Model file for the job. Use its own axes, mm. A direction names the side the tool comes from. Coordinates: 2 decimals unless noted, no trailing zeros. Order: outer loops, then holes, each group sorted by start corner. A loop starts at its lowest first (then second) coordinate and runs counter-clockwise, first axis right, second up.
from build123d import *

# Parameters (mm, degrees)
SKETCH1_W               = 200
SKETCH1_H               = 200
BOSS_EXTRUDE1_DEPTH     = 3
CUT_EXTRUDE1_START      = -4
SKETCH2_W               = 30
SKETCH2_H               = 80
CUT_EXTRUDE1_DEPTH      = 14
FILLET1_R               = 45
SKETCH10_R              = 1.5
CUT_EXTRUDE9_DEPTH      = 4
LPATTERN1_COUNT         = 2
LPATTERN1_PITCH         = 40
LPATTERN1_COUNT_DIR2    = 2
LPATTERN1_PITCH_DIR2    = 20
SKETCH13_R              = 1.5
SKETCH13_W              = 3
SKETCH13_H              = 10
CUT_EXTRUDE10_DEPTH     = 4
SKETCH14_R              = 1.5
CUT_EXTRUDE11_DEPTH     = 4
MIRROR1_COPY_1_SKETCH_R = 1.5
MIRROR1_COPY_1_DEPTH    = 4
MIRROR1_COPY_2_SKETCH_R = 1.5
MIRROR1_COPY_2_DEPTH    = 4
MIRROR1_COPY_3_SKETCH_R = 1.5
MIRROR1_COPY_3_DEPTH    = 4
FILLET2_R               = 0.5
SKETCH23_W              = 60
SKETCH23_H              = 70
CUT_EXTRUDE13_DEPTH     = 10
SKETCH25_W              = 60
SKETCH25_H              = 33
CUT_EXTRUDE15_DEPTH     = 10
SKETCH26_W              = 37.10221973
SKETCH26_H              = 30
BOSS_EXTRUDE3_DEPTH     = 10
SKETCH27_W              = 37
SKETCH27_H              = 27
CUT_EXTRUDE16_DEPTH     = 10
SKETCH30_R              = 2.5
CUT_EXTRUDE17_DEPTH     = 10
SKETCH31_R              = 2.5
CUT_EXTRUDE18_DEPTH     = 10


with BuildPart() as part:
    # Sketch1 → Boss-Extrude1 (new body)
    with BuildSketch(Plane(origin=(0, 0, 0), x_dir=(1, 0, 0), z_dir=(0, 1, 0))):
        Rectangle(SKETCH1_W, SKETCH1_H)
    extrude(amount=BOSS_EXTRUDE1_DEPTH)

    # Sketch2 → Cut-Extrude1 (cut)
    with BuildSketch(Plane(origin=(0, 3, 0), x_dir=(1, 0, 0), z_dir=(0, 1, 0)).offset(CUT_EXTRUDE1_START)):
        with Locations((-85, -40)):
            Rectangle(SKETCH2_W, SKETCH2_H)
    cut_extrude1 = extrude(amount=CUT_EXTRUDE1_DEPTH, mode=Mode.SUBTRACT)

    # Fillet1
    fillet1_edges = [part.edges().sort_by_distance(p)[0] for p in [
        (-100, 1.5, -100),
        (100, 1.5, -100),
    ]]
    fillet(fillet1_edges, radius=FILLET1_R)

    # Sketch10 → Cut-Extrude9 (cut, through all)
    with BuildSketch(Plane(origin=(0, 3, 0), x_dir=(1, 0, 0), z_dir=(0, 1, 0))):
        with Locations((-60, -60)):
            Circle(SKETCH10_R)
    cut_extrude9 = extrude(amount=-CUT_EXTRUDE9_DEPTH, mode=Mode.SUBTRACT)

    # LPattern1: Cut-Extrude9 2 × 2
    with Locations(*[(j * LPATTERN1_PITCH_DIR2, 0, -i * LPATTERN1_PITCH) for i in range(LPATTERN1_COUNT) for j in range(LPATTERN1_COUNT_DIR2) if (i, j) != (0, 0)]):
        add(cut_extrude9, mode=Mode.SUBTRACT)

    # Sketch13 → Cut-Extrude10 (cut, through all)
    with BuildSketch(Plane(origin=(0, 3, 0), x_dir=(1, 0, 0), z_dir=(0, 1, 0))):
        with Locations((-60, 28)):
            Circle(SKETCH13_R)
        with Locations((-40, 35)):
            Rectangle(SKETCH13_W, SKETCH13_H)
    cut_extrude10 = extrude(amount=-CUT_EXTRUDE10_DEPTH, mode=Mode.SUBTRACT)

    # Sketch14 → Cut-Extrude11 (cut, through all)
    with BuildSketch(Plane(origin=(0, 3, 0), x_dir=(1, 0, 0), z_dir=(0, 1, 0))):
        with Locations((-60, -90)):
            Circle(SKETCH14_R)
    cut_extrude11 = extrude(amount=-CUT_EXTRUDE11_DEPTH, mode=Mode.SUBTRACT)

    # Mirror1: Cut-Extrude10, Cut-Extrude9, Cut-Extrude1, Cut-Extrude11 across plane
    add(cut_extrude10.mirror(Plane(origin=(0, 0, 0), x_dir=(0, 0, 1), z_dir=(1, 0, 0))), mode=Mode.SUBTRACT)
    add(cut_extrude9.mirror(Plane(origin=(0, 0, 0), x_dir=(0, 0, 1), z_dir=(1, 0, 0))), mode=Mode.SUBTRACT)
    add(cut_extrude1.mirror(Plane(origin=(0, 0, 0), x_dir=(0, 0, 1), z_dir=(1, 0, 0))), mode=Mode.SUBTRACT)
    add(cut_extrude11.mirror(Plane(origin=(0, 0, 0), x_dir=(0, 0, 1), z_dir=(1, 0, 0))), mode=Mode.SUBTRACT)

    # Mirror1 copy 1 sketch → Mirror1 copy 1 (cut, through all)
    with BuildSketch(Plane(origin=(-20, 3, 0), x_dir=(-1, 0, 0), z_dir=(0, 1, 0))):
        with Locations((-60, 60)):
            Circle(MIRROR1_COPY_1_SKETCH_R)
    extrude(amount=-MIRROR1_COPY_1_DEPTH, mode=Mode.SUBTRACT)

    # Mirror1 copy 2 sketch → Mirror1 copy 2 (cut, through all)
    with BuildSketch(Plane(origin=(0, 3, -40), x_dir=(-1, 0, 0), z_dir=(0, 1, 0))):
        with Locations((-60, 60)):
            Circle(MIRROR1_COPY_2_SKETCH_R)
    extrude(amount=-MIRROR1_COPY_2_DEPTH, mode=Mode.SUBTRACT)

    # Mirror1 copy 3 sketch → Mirror1 copy 3 (cut, through all)
    with BuildSketch(Plane(origin=(-20, 3, -40), x_dir=(-1, 0, 0), z_dir=(0, 1, 0))):
        with Locations((-60, 60)):
            Circle(MIRROR1_COPY_3_SKETCH_R)
    extrude(amount=-MIRROR1_COPY_3_DEPTH, mode=Mode.SUBTRACT)

    # Fillet2
    fillet2_edges = [part.edges().sort_by_distance(p)[0] for p in [
        (100, 3, 90),
        (-100, 0, 90),
        (-100, 3, 90),
        (-70, 3, 40),
        (-70, 0, 40),
        (-85, 3, 0),
        (-85, 0, 0),
        (-85, 3, 80),
        (-85, 0, 80),
        (0, 0, -100),
        (0, 3, -100),
        (-100, 0, -27.5),
        (-86.819805153, 0, -86.819805153),
        (86.819805153, 0, -86.819805153),
        (-100, 3, -27.5),
        (-86.819805153, 3, -86.819805153),
        (86.819805153, 3, -86.819805153),
        (100, 0, 90),
        (0, 0, 100),
        (0, 3, 100),
        (100, 0, -27.5),
        (100, 3, -27.5),
        (70, 3, 40),
        (85, 3, 80),
        (85, 3, 0),
        (70, 0, 40),
        (85, 0, 0),
        (85, 0, 80),
    ]]
    fillet(fillet2_edges, radius=FILLET2_R)

    # Sketch23 → Cut-Extrude13 (cut)
    with BuildSketch(Plane(origin=(0, 3, 0), x_dir=(1, 0, 0), z_dir=(0, 1, 0))):
        with Locations((3.779632889, 35)):
            Rectangle(SKETCH23_W, SKETCH23_H)
    extrude(amount=-CUT_EXTRUDE13_DEPTH, mode=Mode.SUBTRACT)

    # Sketch25 → Cut-Extrude15 (cut)
    with BuildSketch(Plane(origin=(0, 3, 0), x_dir=(1, 0, 0), z_dir=(0, 1, 0))):
        with Locations((3.779632889, 86.5)):
            Rectangle(SKETCH25_W, SKETCH25_H)
    extrude(amount=-CUT_EXTRUDE15_DEPTH, mode=Mode.SUBTRACT)

    # Sketch26 → Boss-Extrude3 (add)
    with BuildSketch(Plane(origin=(0, 3, 0), x_dir=(1, 0, 0), z_dir=(0, 1, 0))):
        with Locations((0, -22)):
            Rectangle(SKETCH26_W, SKETCH26_H)
    extrude(amount=BOSS_EXTRUDE3_DEPTH)

    # Sketch27 → Cut-Extrude16 (cut)
    with BuildSketch(Plane(origin=(0, 3, 0), x_dir=(1, 0, 0), z_dir=(0, 1, 0))):
        with Locations((-44.720367111, 46)):
            Rectangle(SKETCH27_W, SKETCH27_H)
    extrude(amount=-CUT_EXTRUDE16_DEPTH, mode=Mode.SUBTRACT)

    # Sketch30 → Cut-Extrude17 (cut)
    with BuildSketch(Plane(origin=(0, 3, 0), x_dir=(1, 0, 0), z_dir=(0, 1, 0))):
        with Locations((-31.5, -89)):
            Circle(SKETCH30_R)
        with Locations((31.5, -89)):
            Circle(SKETCH30_R)
    extrude(amount=-CUT_EXTRUDE17_DEPTH, mode=Mode.SUBTRACT)

    # Sketch31 → Cut-Extrude18 (cut)
    with BuildSketch(Plane(origin=(0, 3, 0), x_dir=(1, 0, 0), z_dir=(0, 1, 0))):
        with Locations((46, -89)):
            Circle(SKETCH31_R)
    extrude(amount=-CUT_EXTRUDE18_DEPTH, mode=Mode.SUBTRACT)


solid = part.part
Q1. Cut at A-A, the plane x = -50. List the corners of the cut face in (y, z), plus the area to 3 significant figures.
Established:
outline: (0, -99.5) arc R0.5 ccw to (0.5, -100) - (2.5, -100) arc R0.5 ccw to (3, -99.5) - (3, -59.5) - (0, -59.5) - close; (0, -32.5) - (3, -32.5) - (3, 99.5) arc R0.5 ccw to (2.5, 100) - (0.5, 100) arc R0.5 ccw to (0, 99.5) - close
area: 519 mm2
Q2. Cut at C-C, the plane x = -16. List the corners of the cut face in (y, z).
Established:
outline: (0, 0) - (3, 0) - (3, 7) - (13, 7) - (13, 37) - (3, 37) - (3, 99.5) arc R0.5 ccw to (2.5, 100) - (0.5, 100) arc R0.5 ccw to (0, 99.5) - close
Q3. Probe line 1 (X direction, y = 2.2, z = -28); line 2 (Z direction, x = 60, y = 2.35); line 3 (X direction, y = 1.6, z = 89). List the from-to ranges inside material, lowest first.
Established:
line 1: x = -100 to -61.5, -58.5 to -26.22, 33.78 to 58.5, 61.5 to 100
line 2: z = -99.72 to -29.5, -26.5 to 18.5, 21.5 to 58.5, 61.5 to 88.5, 91.5 to 100
line 3: x = -100 to -61.12, -58.88 to -34, -29 to 29, 34 to 43.5, 48.5 to 58.88, 61.12 to 100
Q4. Cut at D-D, the plane x = 31.5. List the corners of the cut face in (y, z), plus the area to 3 significant figures.
Established:
outline: (0, 0) - (3, 0) - (3, 86.5) - (0, 86.5) - close; (0, 91.5) - (3, 91.5) - (3, 99.5) arc R0.5 ccw to (2.5, 100) - (0.5, 100) arc R0.5 ccw to (0, 99.5) - close
area: 285 mm2
Q5. Drop flat-ended pins along their axis: P1, Ø4, axis at x = 60, z = 60, coming from the -Y side; P2, Ø2, axis at x = -90.5, y = 1.5, coming from the -Z side; P3, Ø6, axis at y = 7.5, z = 18.5, coming from the +X side; P4, Ø2, axis at x = 81, y = 1, coming from the -Z side. Give the stop position or say it passes through.
Established:
P1: stops at y = 0
P2: stops at z = -83.89
P3: stops at x = 18.55
P4: stops at z = -92.42
Q6. Mould opens along Z. For faces 1 (the face through (21, 3, 21)), 2 (the face through (0, 8, 37)), 3 (the face through (-31.83, 1.52, 86.52)) say: pulls with the +Z half, pulls with the -Z half, needs draft (parallel to the pull), parting line crosses it, or undercut.
Established:
face 1: needs draft
face 2: pulls with the +Z half
face 3: undercut
Q7. Which spindle directions (+Z, -Z, +X, -X, +Y, -Y) get a long thin tool onto all of the face, cutting with end or side? Do faces 4 (the face through (-18.551, 8, 22)), 5 (the face through (18.551, 8, 22)), 6 (the face through (0, 8, 7)), 7 (the face through (31.17, 1.52, 86.52)). Say none if no direction does.
Established:
face 4: +Z, -Z, -X, +Y
face 5: +Z, -Z, +X, +Y
face 6: -Z, +X, -X, +Y
face 7: +Y, -Y
Q8. Cut at B-B, the plane z = 30. List the corners of the cut face in (x, y), plus the area to 3 significant figures.
Established:
outline: (-70, 0.5) arc R0.5 ccw to (-69.5, 0) - (69.5, 0) arc R0.5 ccw to (70, 0.5) - (70, 2.5) arc R0.5 ccw to (69.5, 3) - (18.55, 3) - (18.55, 13) - (-18.55, 13) - (-18.55, 3) - (-69.5, 3) arc R0.5 ccw to (-70, 2.5) - close
area: 791 mm2
